from build123d import *

# Parameters (mm, degrees)
SKETCH_1_W          = 80
SKETCH_1_H          = 80
SKETCH_1_R          = 26
EXTRUDE_1_DEPTH     = 2
SKETCH_2_R          = 1.5
CUT_EXTRUDE_1_DEPTH = 57.603886792


with BuildPart() as part:
    # 草图1 → 凸台-拉伸1 (new body)
    with BuildSketch(Plane.XY):
        Rectangle(SKETCH_1_W, SKETCH_1_H)
        Circle(SKETCH_1_R, mode=Mode.SUBTRACT)
    extrude(amount=EXTRUDE_1_DEPTH)

    # 草图2 → 切除-拉伸1 (cut, through all)
    with BuildSketch(Plane.XY.offset(2)):
        with Locations((37, 28)):
            Circle(SKETCH_2_R)
        with Locations((37, 18)):
            Circle(SKETCH_2_R)
        with Locations((37, -18)):
            Circle(SKETCH_2_R)
        with Locations((37, -28)):
            Circle(SKETCH_2_R)
        with Locations(Location((-37, -28, 0), (0, 0, 180))):
            Circle(SKETCH_2_R)
        with Locations(Location((-37, -18, 0), (0, 0, 180))):
            Circle(SKETCH_2_R)
        with Locations(Location((-37, 18, 0), (0, 0, 180))):
            Circle(SKETCH_2_R)
        with Locations(Location((-37, 28, 0), (0, 0, 180))):
            Circle(SKETCH_2_R)
        with Locations((-28, 37)):
            Circle(SKETCH_2_R)
        with Locations((-18, 37)):
            Circle(SKETCH_2_R)
        with Locations((18, 37)):
            Circle(SKETCH_2_R)
        with Locations((28, 37)):
            Circle(SKETCH_2_R)
        with Locations(Location((28, -37, 0), (0, 0, 180))):
            Circle(SKETCH_2_R)
        with Locations(Location((18, -37, 0), (0, 0, 180))):
            Circle(SKETCH_2_R)
        with Locations(Location((-18, -37, 0), (0, 0, 180))):
            Circle(SKETCH_2_R)
        with Locations(Location((-28, -37, 0), (0, 0, 180))):
            Circle(SKETCH_2_R)
    extrude(amount=-CUT_EXTRUDE_1_DEPTH, mode=Mode.SUBTRACT)


solid = part.part
Read the model definition and answer for the solid it produces. Units are mm, in the model's axes. Round coordinates to 2 decimals unless told otherwise and drop trailing zeros. Write each loop counter-clockwise with the first axis right and the second up, starting at its lowest first coordinate (ties: lowest second). Pieces come first, ordered by that corner, then holes.
Q1. Find section B-B on x = 0. Determine the outline of the cut face in (y, z).
Values:
outline: (-40, 0) - (-26, 0) - (-26, 2) - (-40, 2) - close; (26, 0) - (40, 0) - (40, 2) - (26, 2) - close
Q2. Find section A-A on y = 10. Determine the outline of the cut face in (x, z).
Values:
outline: (-40, 0) - (-24, 0) - (-24, 2) - (-40, 2) - close; (24, 0) - (40, 0) - (40, 2) - (24, 2) - close
Q3. Find section C-C on y = 28. Determine the outline of the cut face in (x, z).
Values:
outline: (-40, 0) - (-38.5, 0) - (-38.5, 2) - (-40, 2) - close; (-35.5, 0) - (35.5, 0) - (35.5, 2) - (-35.5, 2) - close; (38.5, 0) - (40, 0) - (40, 2) - (38.5, 2) - close
Q4. The mould has two halves that part along Y. Classify faces 1 (the face through (-40, -1, 1)), 2 (the face through (-1, -40, 1)), 3 (the face through (-35.89, 26.99, 1.01)): released by +Y, released by -Y, zero draft, split by the parting line, or undercut.
Values:
face 1: zero draft
face 2: released by -Y
face 3: undercut
Q5. Find section D-D on x = 18. Determine the outline of the cut face in (y, z).
Values:
outline: (-40, 0) - (-38.5, 0) - (-38.5, 2) - (-40, 2) - close; (-35.5, 0) - (-18.76, 0) - (-18.76, 2) - (-35.5, 2) - close; (18.76, 0) - (35.5, 0) - (35.5, 2) - (18.76, 2) - close; (38.5, 0) - (40, 0) - (40, 2) - (38.5, 2) - close
Q6. Straight lines are drawn through the part: line 1 (Y direction, x = 37, z = 0.55); line 2 (Y direction, x = -28, z = 0.5); line 3 (Y direction, x = 18, z = 0.8). For each, find the intervals that lie inside material, in ascending order.
Values:
line 1: y = -40 to -29.5, -26.5 to -19.5, -16.5 to 16.5, 19.5 to 26.5, 29.5 to 40
line 2: y = -40 to -38.5, -35.5 to 35.5, 38.5 to 40
line 3: y = -40 to -38.5, -35.5 to -18.76, 18.76 to 35.5, 38.5 to 40
